Could you check a few things on this model? Use its own coordinates, in mm. Face numbers are marked on the shaded views. A direction names the side the tool comes from. Round coordinates to 2 decimals unless told otherwise and drop trailing zeros. Loops run counter-clockwise (first coordinate to the right, second up) from the corner with the lowest first, then second, coordinate; pieces in that order, holes last. Notation, with made-up numbers: (-19, 10) - (18, 10) arc R17 ccw to (18, 33) - close; hole circle Ø5 at (-37.5, 84.25). An arc over 180 degrees is marked (long way). Use one line per item in the form item = value.
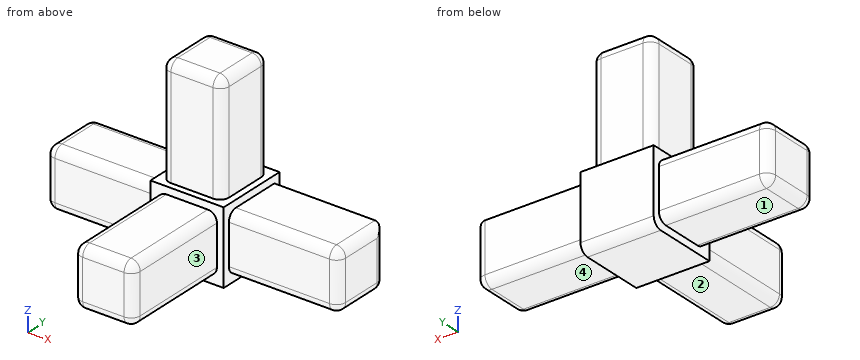
```python
from build123d import *

# Parameters (mm, degrees)
F0_W     = 16.3
F0_H     = 16
F1_DEPTH = 50
F0_W_2   = 20
F0_H_2   = 20
F2_DEPTH = 20
F3_W     = 16.3
F3_H     = 16
F4_DEPTH = 40
F5_W     = 16.3
F5_H     = 16
F6_DEPTH = 40
F7_W     = 16.5
F7_H     = 16.5
F8_DEPTH = 40
F9_R     = 2.5


with BuildPart() as f1:
    # F0 (on Front) → F1 (new body)
    with BuildSketch(Plane.XZ):
        Rectangle(F0_W, F0_H)
    extrude(amount=F1_DEPTH)

    # F0 (on Front) → F2 (join)
    with BuildSketch(Plane.XZ):
        Rectangle(F0_W_2, F0_H_2)
        Rectangle(F0_W, F0_H, mode=Mode.SUBTRACT)
    extrude(amount=F2_DEPTH)

    # F3 (on Right) → F4 (join)
    with BuildSketch(Plane.YZ):
        with Locations((-10, 0)):
            Rectangle(F3_W, F3_H)
    extrude(amount=F4_DEPTH)

    # F5 (on Right) → F6 (join)
    with BuildSketch(Plane.YZ):
        with Locations((-10, 0)):
            Rectangle(F5_W, F5_H)
    extrude(amount=-F6_DEPTH)

    # F7 (on Top) → F8 (join)
    with BuildSketch(Plane.XY):
        with Locations((0, -10)):
            Rectangle(F7_W, F7_H)
    extrude(amount=F8_DEPTH)

    # F9
    f9_edges = [f1.edges().sort_by_distance(p)[0] for p in [
        (0, 0, -10),
        (-25, -1.85, -8),
        (-25, -18.15, -8),
        (-25, -1.85, 8),
        (-25, -18.15, 8),
        (-40, -10, -8),
        (-40, -1.85, 0),
        (-40, -10, 8),
        (-40, -18.15, 0),
        (-8.25, -18.25, 25),
        (0, -18.25, 40),
        (-8.25, -10, 40),
        (8.25, -10, 40),
        (0, -1.75, 40),
        (-8.25, -1.75, 25),
        (8.25, -1.75, 25),
        (8.25, -18.25, 25),
        (-8.15, -35, 8),
        (0, -50, 8),
        (8.15, -35, 8),
        (-8.15, -50, 0),
        (0, -50, -8),
        (8.15, -50, 0),
        (25, -18.15, 8),
        (25, -18.15, -8),
        (40, -10, -8),
        (40, -1.85, 0),
        (40, -10, 8),
        (40, -18.15, 0),
        (8.15, -35, -8),
        (-8.15, -35, -8),
        (25, -1.85, -8),
    ]]
    fillet(f9_edges, radius=F9_R)


solid = f1.part
```
1. Please list where these lines run through material, in increasing order: line 1 along X through (y, z) = (-21.5, -1.5); line 2 along Y through (x, z) = (6, 25); line 3 along Z through (x, y) = (20, -6).
Solution:
line_1 = -8.15 to 8.15
line_2 = -18.24 to -1.76
line_3 = -8 to 8
2. If we section it at B-B, the plane z = 15: Write out the boundary of the cut face in (x, y), plus the area to 3 significant figures.
Solution:
outline = (-8.25, -15.75) arc R2.5 ccw to (-5.75, -18.25) - (5.75, -18.25) arc R2.5 ccw to (8.25, -15.75) - (8.25, -4.25) arc R2.5 ccw to (5.75, -1.75) - (-5.75, -1.75) arc R2.5 ccw to (-8.25, -4.25) - close
area = 267 mm^2
3. On a 3-axis mill with a long thin cutter (end or side, diameter ignored), from which of +Z, -Z, +X, -X, +Y, -Y can I reach the whole of each face in a straight line? I mean the marked faces 1, 2, 3 and 4. Say none if no direction works.
Solution:
face_1 = -Z, -X, +Y, -Y
face_2 = -Z, +X, -X, -Y
face_3 = +Z, -Z, +X, -Y
face_4 = -Z, +X, +Y, -Y
4. If we section it at D-D, the plane x = 11.5: Write out the boundary of the cut face in (y, z), plus the area to 3 significant figures.
Solution:
outline = (-18.15, -5.5) arc R2.5 ccw to (-15.65, -8) - (-4.35, -8) arc R2.5 ccw to (-1.85, -5.5) - (-1.85, 8) - (-15.65, 8) arc R2.5 ccw to (-18.15, 5.5) - close
area = 257 mm^2
5. If we section it at A-A, the plane x = -4: Write out the boundary of the cut face in (y, z), plus the area to 3 significant figures.
Solution:
outline = (-50, -5.5) arc R2.5 ccw to (-47.5, -8) - (-20, -8) - (-20, -10) - (-2.5, -10) arc R2.5 ccw to (0, -7.5) - (0, 10) - (-1.75, 10) - (-1.75, 37.5) arc R2.5 ccw to (-4.25, 40) - (-15.75, 40) arc R2.5 ccw to (-18.25, 37.5) - (-18.25, 10) - (-20, 10) - (-20, 8) - (-47.5, 8) arc R2.5 ccw to (-50, 5.5) - close
area = 1,370 mm^2
6. If we section it at C-C, the plane y = -9: Write out the boundary of the cut face in (x, z), plus the area to 3 significant figures.
Solution:
outline = (-40, -5.5) arc R2.5 ccw to (-37.5, -8) - (-10, -8) - (-10, -10) - (10, -10) - (10, -8) - (37.5, -8) arc R2.5 ccw to (40, -5.5) - (40, 5.5) arc R2.5 ccw to (37.5, 8) - (10, 8) - (10, 10) - (8.25, 10) - (8.25, 37.5) arc R2.5 ccw to (5.75, 40) - (-5.75, 40) arc R2.5 ccw to (-8.25, 37.5) - (-8.25, 10) - (-10, 10) - (-10, 8) - (-37.5, 8) arc R2.5 ccw to (-40, 5.5) - close
area = 1,850 mm^2
7. For P1, Ø12.5, axis at x = 24.5, y = -9, coming from the -Z side; P2, Ø3.5, axis at x = -1, z = 28.5, coming from the +Y side; P3, Ø10, axis at x = 27, z = -5, coming from the -Y side, each with a flat end and sliding along its axis, tell me the tip position at first contact or that it passes through.
Solution:
P1 = -8
P2 = -1.75
P3 = -18.15
